```python
from build123d import *

# Parameters (mm, degrees)
SKETCH1_W           = 97.5
SKETCH1_H           = 97.5
BOSS_EXTRUDE1_DEPTH = 0.8
SKETCH2_W           = 7.6
SKETCH2_H           = 7.6
CUT_EXTRUDE1_DEPTH  = 1.8
SKETCH3_R           = 1.7
CUT_EXTRUDE2_DEPTH  = 1.8
CUT_EXTRUDE3_DEPTH  = 1.8
SKETCH5_R           = 0.5
CUT_EXTRUDE4_DEPTH  = 1.8
FILLET2_R           = 3


with BuildPart() as part:
    # Sketch1 → Boss-Extrude1 (new body)
    with BuildSketch(Plane.XY):
        Rectangle(SKETCH1_W, SKETCH1_H)
    extrude(amount=BOSS_EXTRUDE1_DEPTH)

    # Sketch2 → Cut-Extrude1 (cut, through all)
    with BuildSketch(Plane(origin=(0, 0, 0), x_dir=(-1, 0, 0), z_dir=(0, 0, -1))):
        with Locations((-44.95, 44.95)):
            Rectangle(SKETCH2_W, SKETCH2_H)
        with Locations((-44.95, -44.95)):
            Rectangle(SKETCH2_W, SKETCH2_H)
        with Locations((44.95, -44.95)):
            Rectangle(SKETCH2_W, SKETCH2_H)
        with Locations((44.95, 44.95)):
            Rectangle(SKETCH2_W, SKETCH2_H)
    extrude(amount=-CUT_EXTRUDE1_DEPTH, mode=Mode.SUBTRACT)

    # Sketch3 → Cut-Extrude2 (cut, through all)
    with BuildSketch(Plane(origin=(0, 0, 0), x_dir=(-1, 0, 0), z_dir=(0, 0, -1))):
        with Locations((0, 35.2)):
            Circle(SKETCH3_R)
        with Locations((35.2, 0)):
            Circle(SKETCH3_R)
        with Locations((0, -35.2)):
            Circle(SKETCH3_R)
        with Locations((-35.2, 0)):
            Circle(SKETCH3_R)
    extrude(amount=-CUT_EXTRUDE2_DEPTH, mode=Mode.SUBTRACT)

    # Sketch4 → Cut-Extrude3 (cut, through all)
    with BuildSketch(Plane(origin=(0, 0, 0), x_dir=(-1, 0, 0), z_dir=(0, 0, -1))):
        Polygon((-18.03122292, 12.374368671), (-13.717871555, 8.061017306), (-8.061017306, 13.717871555), (-12.374368671, 18.03122292), align=None)
    extrude(amount=-CUT_EXTRUDE3_DEPTH, mode=Mode.SUBTRACT)

    # Sketch5 → Cut-Extrude4 (cut, through all)
    with BuildSketch(Plane(origin=(0, 0, 0), x_dir=(-1, 0, 0), z_dir=(0, 0, -1))):
        with Locations((-6.965001795, 13.682516216)):
            Circle(SKETCH5_R)
        with Locations((-5.833630945, 12.551145366)):
            Circle(SKETCH5_R)
        with Locations((-8.485281374, 8.485281374)):
            Circle(SKETCH5_R)
        with Locations((-7.353910524, 7.353910524)):
            Circle(SKETCH5_R)
        with Locations((-10.005560954, 3.288046533)):
            Circle(SKETCH5_R)
        with Locations((-8.874190104, 2.156675683)):
            Circle(SKETCH5_R)
    extrude(amount=-CUT_EXTRUDE4_DEPTH, mode=Mode.SUBTRACT)

    # Fillet2
    fillet2_edges = [part.edges().sort_by_distance(p)[0] for p in [
        (18.03122292, 12.374368671, 0.4),
        (12.374368671, 18.03122292, 0.4),
        (8.061017306, 13.717871555, 0.4),
        (13.717871555, 8.061017306, 0.4),
    ]]
    fillet(fillet2_edges, radius=FILLET2_R)


solid = part.part
```
Design review of the part built by this model. Coordinates are the model's own, in mm. Round coordinates to 2 decimals unless told otherwise and drop trailing zeros. Write each loop counter-clockwise with the first axis right and the second up, starting at its lowest first coordinate (ties: lowest second). Pieces come first, ordered by that corner, then holes.
Item 1: We need section A-A on y = 0. Write out the cut boundary in (x, z), and give its area (3 significant figures).
Item 2: We need section C-C on y = -35.2. Write out the cut boundary in (x, z).
Item 3: For probe 1 along Y at (x, z) = (0, 0.25); probe 2 along Y at (x, z) = (-35.2, 0.5); probe 3 along X at (y, z) = (-41.5, 0.2), list the stretches that pass through material, from the lowest coordinate up.
Item 4: The part is to be moulded in two halves that separate along X. For faces 1 (the flat face through (-1, 1, 0)), 2 (the cylindrical face through (1.35, -36.23, 0.39)), 3 (the cylindrical face through (33.58, 0.51, 0.39)), say which applies: +X half, -X half, draft (parallel to the pull), parting line (faces both ways), or undercut.
Returned:
1. outline: (-48.75, 0) - (-36.9, 0) - (-36.9, 0.8) - (-48.75, 0.8) - close; (-33.5, 0) - (33.5, 0) - (33.5, 0.8) - (-33.5, 0.8) - close; (36.9, 0) - (48.75, 0) - (48.75, 0.8) - (36.9, 0.8) - close
1. area: 72.6 mm2
2. outline: (-48.75, 0) - (-1.7, 0) - (-1.7, 0.8) - (-48.75, 0.8) - close; (1.7, 0) - (48.75, 0) - (48.75, 0.8) - (1.7, 0.8) - close
3. probe 1: y = -48.75 to -36.9, -33.5 to 33.5, 36.9 to 48.75
3. probe 2: y = -48.75 to -1.7, 1.7 to 48.75
3. probe 3: x = -41.15 to 41.15
4. face 1: draft
4. face 2: undercut
4. face 3: undercut
